Could you check a few things on this drawing? It's one solid part, dimensions in mm from its lowest x, y, z. A direction names the side the tool comes from. Coordinates: 2 decimals unless noted, no trailing zeros. Order: outer loops, then holes, each group sorted by start corner. A loop starts at its lowest first (then second) coordinate and runs counter-clockwise, first axis right, second up. Notation, with made-up numbers: (84, 69) -> (101, 69) arc R30 ccw to (101, 95) -> close; hole circle Ø9 at (85, 38). An arc over 180 degrees is marked (long way). Use a Markdown table: item, result. Add a question column.
1. Suppose I cut it at D-D, the plane x = 15.25. List the corners of the cut face in (y, z) for me.
2. For pin 1 Ø0.6 at (x, z) = (1.5, 1) entering from +Y; pin 2 Ø0.6 at (y, z) = (16, 0.5) entering from -X; pin 3 Ø0.6 at (x, z) = (1, 0.5) entering from -Y, each with a flat end and sliding along its axis, tell me the tip position at first contact or that it passes through.
3. Suppose I cut it at A-A, the plane y = 19.24. List the corners of the cut face in (x, z) for me, then the cut area to 3 significant figures.
4. If I drill on line 1 along Y through (x, z) = (13.45, 0.7); line 2 along X through (y, z) = (19.25, 1.55); line 3 along Y through (x, z) = (15, 1.25), over which ranges is the centre line in solid material (lowest first)? Write a range as from..to.
5. Suppose I cut it at B-B, the plane z = 1.5. List the corners of the cut face in (x, y) for me.
6. Suppose I cut it at C-C, the plane x = 13.45. List the corners of the cut face in (y, z) for me, then the cut area to 3 significant figures.
7. For the marked faces 1, 2 and 3, which set-ups out of +Z, -Z, +X, -X, +Y, -Y let a thin tool reach every point of the face, with its end or its side?
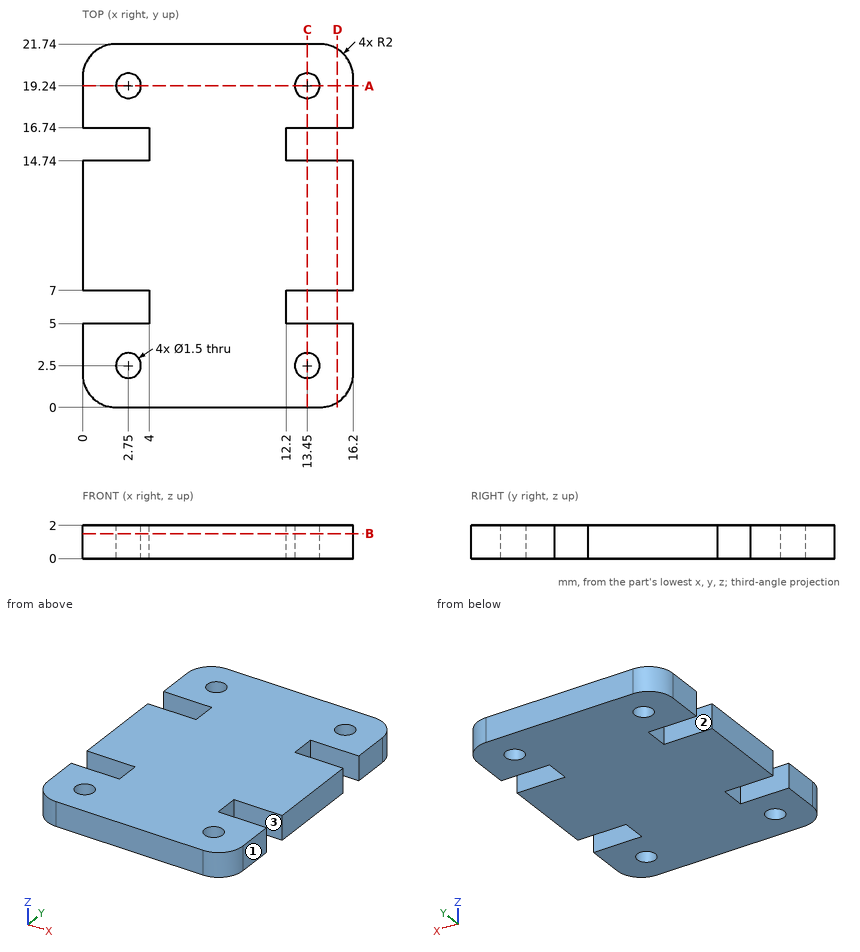
Worked out:
| question | item | result |
|---|---|---|
| 1 | outline | (0.3, 0) -> (5, 0) -> (5, 2) -> (0.3, 2) -> close; (7, 0) -> (14.74, 0) -> (14.74, 2) -> (7, 2) -> close; (16.74, 0) -> (21.44, 0) -> (21.44, 2) -> (16.74, 2) -> close |
| 2 | pin 1 | stops at y = 21.73 |
| 2 | pin 2 | stops at x = 4 |
| 2 | pin 3 | stops at y = 0.13 |
| 3 | outline | (0, 0) -> (2, 0) -> (2, 2) -> (0, 2) -> close; (3.5, 0) -> (12.7, 0) -> (12.7, 2) -> (3.5, 2) -> close; (14.2, 0) -> (16.2, 0) -> (16.2, 2) -> (14.2, 2) -> close |
| 3 | area | 26.4 mm² |
| 4 | line 1 | y = 0..1.75, 3.25..5, 7..14.74, 16.74..18.49, 19.99..21.74 |
| 4 | line 2 | x = 0..2, 3.5..12.7, 14.2..16.2 |
| 4 | line 3 | y = 0.17..5, 7..14.74, 16.74..21.57 |
| 5 | outline | (0, 2) arc R2 ccw to (2, 0) -> (14.2, 0) arc R2 ccw to (16.2, 2) -> (16.2, 5) -> (12.2, 5) -> (12.2, 7) -> (16.2, 7) -> (16.2, 14.74) -> (12.2, 14.74) -> (12.2, 16.74) -> (16.2, 16.74) -> (16.2, 19.74) arc R2 ccw to (14.2, 21.74) -> (2, 21.74) arc R2 ccw to (0, 19.74) -> (0, 16.74) -> (4, 16.74) -> (4, 14.74) -> (0, 14.74) -> (0, 7) -> (4, 7) -> (4, 5) -> (0, 5) -> close; hole circle Ø1.5 at (2.75, 2.5); hole circle Ø1.5 at (2.75, 19.24); hole circle Ø1.5 at (13.45, 2.5); hole circle Ø1.5 at (13.45, 19.24) |
| 6 | outline | (0, 0) -> (1.75, 0) -> (1.75, 2) -> (0, 2) -> close; (3.25, 0) -> (5, 0) -> (5, 2) -> (3.25, 2) -> close; (7, 0) -> (14.74, 0) -> (14.74, 2) -> (7, 2) -> close; (16.74, 0) -> (18.49, 0) -> (18.49, 2) -> (16.74, 2) -> close; (19.99, 0) -> (21.74, 0) -> (21.74, 2) -> (19.99, 2) -> close |
| 6 | area | 29.5 mm² |
| 7 | face 1 | +Z, -Z, +X, +Y, -Y |
| 7 | face 2 | +Z, -Z, -X |
| 7 | face 3 | +Z, -Z, +X |
